Source: CAD feature listing. Evaluate the final solid. Frame: model axes, mm. A direction names the side the tool comes from. Coordinates: 2 decimals unless noted, no trailing zeros. Order: outer loops, then holes, each group sorted by start corner. A loop starts at its lowest first (then second) coordinate and runs counter-clockwise, first axis right, second up.
```python
from build123d import *

# Parameters (mm, degrees)
SKETCH1_W           = 75
SKETCH1_H           = 75
BOSS_EXTRUDE1_DEPTH = 28
SKETCH2_W           = 71
SKETCH2_H           = 71
CUT_EXTRUDE1_DEPTH  = 29
SKETCH3_W           = 10
SKETCH3_H           = 6
CUT_EXTRUDE2_DEPTH  = 2
SKETCH4_W           = 15
SKETCH4_H           = 14
CUT_EXTRUDE3_DEPTH  = 76
SKETCH5_W           = 6
SKETCH5_H           = 15
CUT_EXTRUDE4_DEPTH  = 2


with BuildPart() as part:
    # Sketch1 → Boss-Extrude1 (new body)
    with BuildSketch(Plane(origin=(0, 0, 0), x_dir=(1, 0, 0), z_dir=(0, 1, 0))):
        Rectangle(SKETCH1_W, SKETCH1_H)
    extrude(amount=BOSS_EXTRUDE1_DEPTH)

    # Sketch2 → Cut-Extrude1 (cut, through all)
    with BuildSketch(Plane(origin=(0, 28, 0), x_dir=(1, 0, 0), z_dir=(0, 1, 0))):
        Rectangle(SKETCH2_W, SKETCH2_H)
    extrude(amount=-CUT_EXTRUDE1_DEPTH, mode=Mode.SUBTRACT)

    # Sketch3 → Cut-Extrude2 (cut)
    with BuildSketch(Plane.XY.offset(37.5)):
        with Locations((-17.5, 13)):
            Rectangle(SKETCH3_W, SKETCH3_H)
        Polygon((-6.5, 24), (6.5, 24), (6.5, 21), (9.5, 21), (9.5, 10), (-9.5, 10), (-9.5, 21), (-6.5, 21), align=None)
    extrude(amount=-CUT_EXTRUDE2_DEPTH, mode=Mode.SUBTRACT)

    # Sketch4 → Cut-Extrude3 (cut, through all)
    with BuildSketch(Plane.ZY.offset(37.5)):
        Polygon((12.5, 23), (24.5, 23), (24.5, 20), (27.5, 20), (27.5, 10), (9.5, 10), (9.5, 20), (12.5, 20), align=None)
        with Locations((-23, 7)):
            Rectangle(SKETCH4_W, SKETCH4_H)
    extrude(amount=-CUT_EXTRUDE3_DEPTH, mode=Mode.SUBTRACT)

    # Sketch5 → Cut-Extrude4 (cut)
    with BuildSketch(Plane(origin=(0, 0, -37.5), x_dir=(-1, 0, 0), z_dir=(0, 0, -1))):
        with Locations((2.5, 7.5)):
            Rectangle(SKETCH5_W, SKETCH5_H)
    extrude(amount=-CUT_EXTRUDE4_DEPTH, mode=Mode.SUBTRACT)


solid = part.part
```
Q1. Material intervals for line 1 along Z through (x, y) = (13, 1.5); line 2 along Z through (x, y) = (0, 18.5), sorted ascending.
Solutions:
line 1: z = -37.5 to -35.5, 35.5 to 37.5
line 2: z = -37.5 to -35.5
Q2. Section query B-B on y = 22. Output: boundary loops of the cut face in (x, z).
Solutions:
outline: (-37.5, -37.5) - (37.5, -37.5) - (37.5, 12.5) - (35.5, 12.5) - (35.5, -35.5) - (-35.5, -35.5) - (-35.5, 12.5) - (-37.5, 12.5) - close; (-37.5, 24.5) - (-35.5, 24.5) - (-35.5, 35.5) - (-6.5, 35.5) - (-6.5, 37.5) - (-37.5, 37.5) - close; (6.5, 35.5) - (35.5, 35.5) - (35.5, 24.5) - (37.5, 24.5) - (37.5, 37.5) - (6.5, 37.5) - close
Q3. Section query C-C on x = -2.5. Output: boundary loops of the cut face in (y, z).
Solutions:
outline: (0, 35.5) - (10, 35.5) - (10, 37.5) - (0, 37.5) - close; (15, -37.5) - (28, -37.5) - (28, -35.5) - (15, -35.5) - close; (24, 35.5) - (28, 35.5) - (28, 37.5) - (24, 37.5) - close
Q4. Set-up query: faces 1 (the flat face through (-18, 16, 37)), 2 (the flat face through (36, 7, -15.5)), 3 (the flat face through (35.5, 14, 0)), 4 (the flat face through (36, 15, 9.5)). Return all of +Z, -Z, +X, -X, +Y, -Y with unobstructed straight access to the full face (end or side cutting, diameter ignored); none if empty.
Solutions:
face 1: +Z
face 2: +X, -X, -Y
face 3: +Y, -Y
face 4: +X, -X
Q5. Section query D-D on z = 17.5. Output: boundary loops of the cut face in (x, y), plus the area to 3 significant figures.
Solutions:
outline: (-37.5, 0) - (-35.5, 0) - (-35.5, 10) - (-37.5, 10) - close; (-37.5, 23) - (-35.5, 23) - (-35.5, 28) - (-37.5, 28) - close; (35.5, 0) - (37.5, 0) - (37.5, 10) - (35.5, 10) - close; (35.5, 23) - (37.5, 23) - (37.5, 28) - (35.5, 28) - close
area: 60.0 mm2
Q6. Pull-direction query (Y, two-part tool) for faces 5 (the flat face through (-25, 0, -36)), 6 (the flat face through (-37, 7, -15.5)), 7 (the flat face through (0, 10, 37)), 8 (the flat face through (-18, 10, 37)); classes: pulls with the +Y half, pulls with the -Y half, needs draft (parallel to the pull), parting line crosses it, or undercut.
Solutions:
face 5: pulls with the -Y half
face 6: needs draft
face 7: undercut
face 8: undercut
Q7. Pin query (flat end, axial travel): P1, Ø1, axis at x = -36, z = -24.5, coming from the -Y side. Return the tip coordinate at first contact, or that it passes through.
Solutions:
P1: stops at y = 14
Q8. Section query A-A on z = -22.5. Output: boundary loops of the cut face in (x, y).
Solutions:
outline: (-37.5, 14) - (-35.5, 14) - (-35.5, 28) - (-37.5, 28) - close; (35.5, 14) - (37.5, 14) - (37.5, 28) - (35.5, 28) - close
